For this review, take the finished solid that the model builds, in its own axes (mm). Coordinates: 2 decimals unless noted, no trailing zeros. Write each loop counter-clockwise with the first axis right and the second up, starting at its lowest first coordinate (ties: lowest second). Pieces come first, ordered by that corner, then holes. Notation, with made-up numbers: (13, 30.5) - (47, 30.5) arc R16 ccw to (47, 38.5) - close; hole circle Ø2 at (-27, 36). An arc over 180 degrees is marked (long way). Write each question's results on one line, items separated by ' | '.
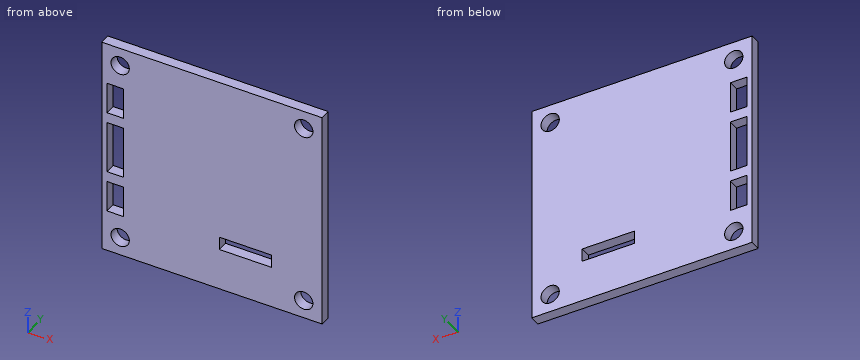
Autodesk Inventor part; units mm, degrees
ref_plane "YZ Plane" through (0, 0, 0) normal (1, 0, 0) x (0, 1, 0)
ref_plane "XZ Plane" through (0, 0, 0) normal (0, 1, 0) x (-1, 0, 0)
ref_plane "XY Plane" through (0, 0, 0) normal (0, 0, 1) x (1, 0, 0)
ref_plane "Work Plane1" through (0, -2.5, 0) normal (0, 1, 0) x (1, 0, 0)
sketch "Sketch10" plane through (0, -2.5, 0) normal (0, 1, 0) x (1, 0, 0)
  line L0 (-24.3453, 76.929) -> (17.6547, 76.929)
  line L1 (17.6547, 76.929) -> (17.6547, 34.929)
  line L2 (17.6547, 34.929) -> (-24.3453, 34.929)
  line L3 (-24.3453, 34.929) -> (-24.3453, 76.929)
  circle A0 centre (-20.8453, 73.429) radius 1.75
  circle A1 centre (14.1547, 73.429) radius 1.75
  circle A2 centre (14.1547, 38.429) radius 1.75
  circle A3 centre (-20.8453, 38.429) radius 1.75
  line L4 (-23.3453, 68.929) -> (-20.1928, 68.929)
  line L5 (-20.1928, 68.929) -> (-20.1928, 42.929)
  line L6 (-20.1928, 42.929) -> (-23.3453, 42.929)
  line L7 (-24.3453, 42.929) -> (-24.3453, 68.9078)
  line L8 (-1.9453, 68.929) -> (8.0547, 68.929)
  line L9 (8.0547, 68.929) -> (8.0547, 66.429)
  line L10 (8.0547, 66.429) -> (-1.9453, 66.429)
  line L11 (-1.9453, 66.429) -> (-1.9453, 68.929)
  line L12 (-23.3453, 62.929) -> (-20.1928, 62.929)
  line L13 (-20.1928, 62.929) -> (-20.1928, 60.929)
  line L14 (-20.1928, 60.929) -> (-23.3453, 60.929)
  line L15 (-23.3453, 50.929) -> (-20.1928, 50.929)
  line L16 (-20.1928, 50.929) -> (-20.1928, 48.929)
  line L17 (-20.1928, 48.929) -> (-23.3453, 48.929)
  line L18 (-23.3453, 68.929) -> (-23.3453, 62.929)
  line L19 (-23.3453, 60.929) -> (-23.3453, 50.929)
  line L20 (-23.3453, 48.929) -> (-23.3453, 42.929)
  point P0 (0, 0)
  point P1 (8.0547, 67.679)
  point P2 (-21.769, 68.929)
  point P3 (-21.769, 62.929)
  point P4 (-21.769, 48.929)
  point P5 (-21.769, 50.929)
  point P6 (-21.769, 42.929)
  dimension "d76" = 42
  dimension "d77" = 42
  dimension "d78" = 3.5
  dimension "d79" = 3.5
  dimension "d80" = 3.5
  dimension "d81" = 3.5
  dimension "d82" = 3.5
  dimension "d83" = 3.5
  dimension "d84" = 3.5
  dimension "d85" = 3.5
  dimension "d86" = 3.5
  dimension "d88" = 10
  dimension "d89" = 2.5
  dimension "d90" = 8
  dimension "d91" = 9.6
  dimension "d92" = 6
  dimension "d93" = 2
  dimension "d94" = 2
  dimension "d95" = 6
  dimension "d96" = 8
  dimension "d97" = 8
extrude "Extrusion9" add sketch "Sketch10" along normal blind 2
equation "\"d80\" = d79"
equation "\"d81\" = d80"
equation "\"d82\" = d80"
equation "\"d83\" = d80"
equation "\"d84\" = d83"
equation "\"d85\" = d80"
equation "\"d86\" = d80"
properties part number "display_base"
Q1. Take a section at A-A on z = -52.5. State the section outline as (x, y) points, plus the area to 3 significant figures.
Results found:
outline: (-24.35, -2.5) - (-23.35, -2.5) - (-23.35, -0.5) - (-24.35, -0.5) - close; (-20.19, -2.5) - (17.65, -2.5) - (17.65, -0.5) - (-20.19, -0.5) - close | area: 77.7 mm2
Q2. For pin 1 (3 mm diameter, centred on x = 14.15, z = -38.43, fed in from +Y), flat-tipped, find the tip position at first contact; note if it passes through.
Results found:
pin 1: through
Q3. Wall thickness on line 1 along X through (y, z) = (-1.05, -60); line 2 along Z through (x, y) = (2, -1.7); line 3 along Z through (x, y) = (13, -2.05): over which ranges is each line inside the solid? List them lowest first. Write a range as from..to.
Results found:
line 1: -24.35..-23.35, -20.19..17.65 | line 2: -76.93..-68.93, -66.43..-34.93 | line 3: -76.93..-74.74, -72.11..-39.74, -37.11..-34.93
Q4. Take a section at D-D on x = 14. State the section outline as (y, z) points, plus the area to 3 significant figures.
Results found:
outline: (-2.5, -76.93) - (-0.5, -76.93) - (-0.5, -75.17) - (-2.5, -75.17) - close; (-2.5, -71.69) - (-0.5, -71.69) - (-0.5, -40.17) - (-2.5, -40.17) - close; (-2.5, -36.69) - (-0.5, -36.69) - (-0.5, -34.93) - (-2.5, -34.93) - close | area: 70.1 mm2
Q5. Take a section at C-C on y = -1.35. State how many separate pieces and enclosed holes the cut face has, plus the area to 3 significant figures.
Results found:
separate pieces: 1 | enclosed holes: 8 | area: 1,630 mm2
Q6. Take a section at B-B on x = 4.5. State the section outline as (y, z) points.
Results found:
outline: (-2.5, -76.93) - (-0.5, -76.93) - (-0.5, -68.93) - (-2.5, -68.93) - close; (-2.5, -66.43) - (-0.5, -66.43) - (-0.5, -34.93) - (-2.5, -34.93) - close
